Answer from the drawing. Dimensions are ordinates in mm from the lowest x, y and z of the part. A direction names the side the tool comes from. Give positions to 0.01 mm unless a question says otherwise; leave off trailing zeros. Order: outer loops, then holes, each group sorted by start corner. A loop starts at its lowest first (then second) coordinate and runs counter-clockwise, first axis right, second up.
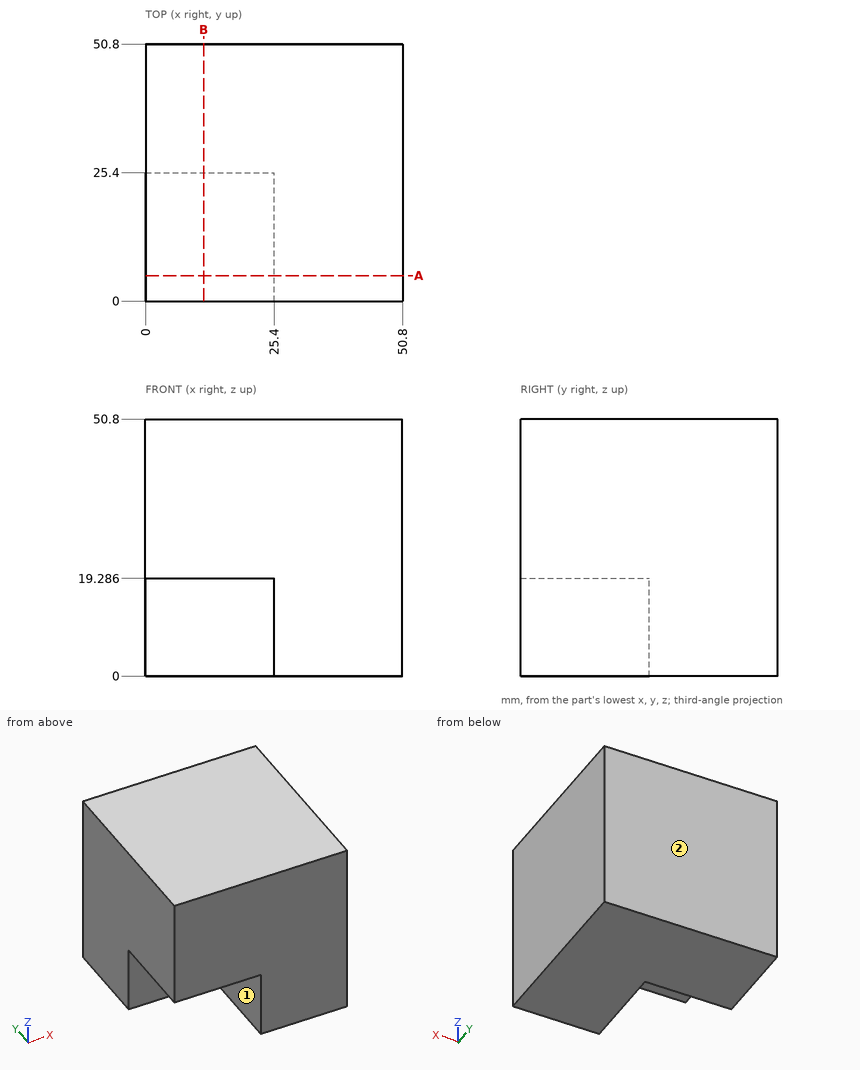
1) Given pin 1 (1.5 mm diameter, centred on x = 24.5, y = 29.5, fed in from -Z); pin 2 (7.5 mm diameter, centred on x = 14, y = 7.5, fed in from -Z); pin 3 (3 mm diameter, centred on x = 19.5, z = 17.5, fed in from -Y); pin 4 (6 mm diameter, centred on y = 15, z = 6, fed in from -X), each flat-ended and moving along its own axis, determine where each tip first touches the part or whether it passes through.
Final values:
pin 1: stops at z = 0
pin 2: stops at z = 19.29
pin 3: stops at y = 25.4
pin 4: stops at x = 25.4
2) A tool of negligible diameter and unlimited length cuts with its end or side. For the marked faces 1 and 2, from which of +Z, -Z, +X, -X, +Y, -Y can it reach the whole face along a straight path? Write none if from no direction.
Final values:
face 1: -Z, -X, -Y
face 2: +Z, -Z, +X, -X, +Y
3) The part is cut by section A-A on y = 5. Determine the outline of the cut face in (x, z), and give its area (3 significant figures).
Final values:
outline: (0, 19.29) - (25.4, 19.29) - (25.4, 0) - (50.8, 0) - (50.8, 50.8) - (0, 50.8) - close
area: 2,090 mm2
4) Consider L1, parallel to Z at x = 25, y = 7; L2, parallel to X at y = 6, z = 16. Determine where each line is inside the solid, lowest interval first.
Final values:
L1: z = 19.29 to 50.8
L2: x = 25.4 to 50.8
